Verification items for this drawing (mm, ordinates from the low corner). Coordinates: 2 decimals unless noted, no trailing zeros. Order: outer loops, then holes, each group sorted by start corner. A loop starts at its lowest first (then second) coordinate and runs counter-clockwise, first axis right, second up.
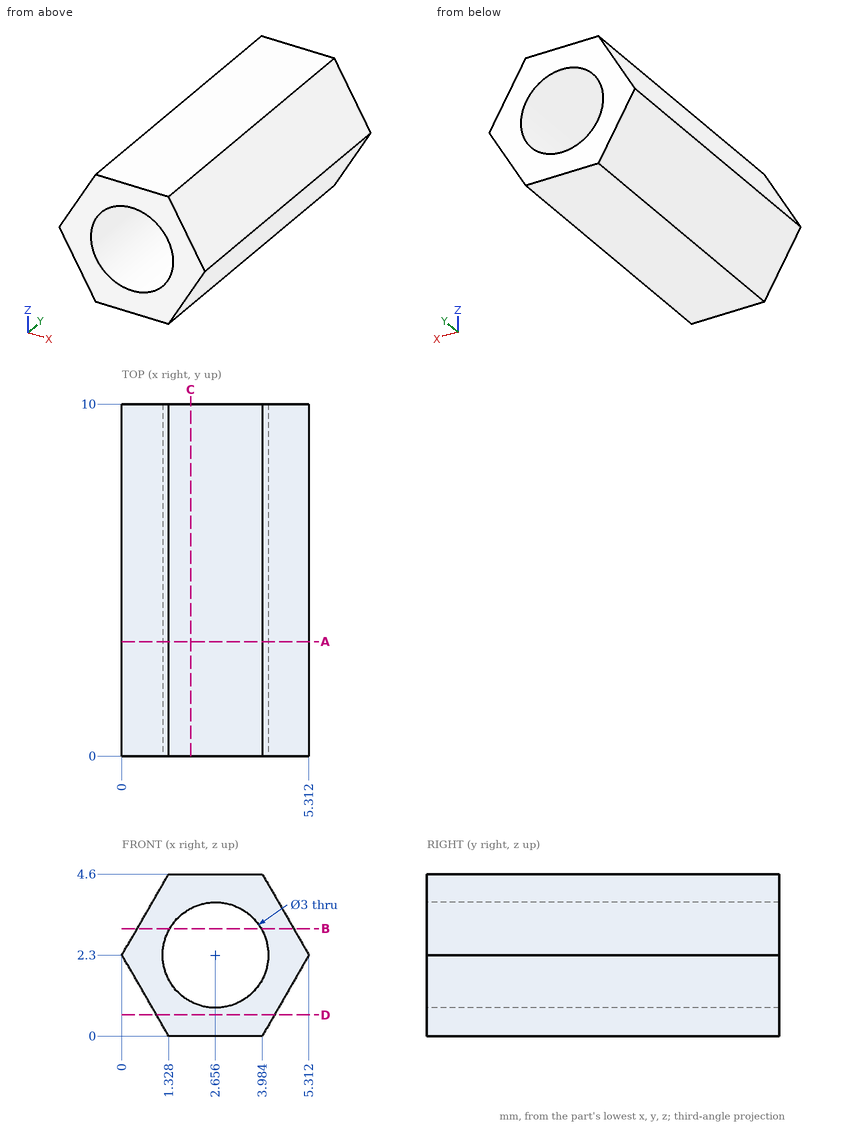
Item 1: Sectioned sample at D-D (z = 0.6). Record the cut outline in (x, y).
Item 2: Thickness scan on line 1 along Z through (x, y) = (2, 3.75); line 2 along Z through (x, y) = (3.5, 4); line 3 along X through (y, z) = (5.5, 1.25) (1 decimal). Record the ranges inside material, lowest first.
Item 3: Sectioned sample at B-B (z = 3.05). Record the cut outline in (x, y) (1 decimal).
Item 4: Sectioned sample at C-C (x = 1.95). Record the cut outline in (y, z).
Item 5: Sectioned sample at A-A (y = 3.25). Record the cut outline in (x, z).
Geometry check:
1. outline: (0.98, 0) - (4.33, 0) - (4.33, 10) - (0.98, 10) - close
2. line 1: z = 0 to 0.95, 3.65 to 4.6
2. line 2: z = 0 to 1.06, 3.54 to 4.6
2. line 3: x = 0.6 to 1.6, 3.7 to 4.7
3. outline: (0.4, 0) - (1.4, 0) - (1.4, 10) - (0.4, 10) - close; (4, 0) - (4.9, 0) - (4.9, 10) - (4, 10) - close
4. outline: (0, 0) - (10, 0) - (10, 0.98) - (0, 0.98) - close; (0, 3.62) - (10, 3.62) - (10, 4.6) - (0, 4.6) - close
5. outline: (0, 2.3) - (1.33, 0) - (3.98, 0) - (5.31, 2.3) - (3.98, 4.6) - (1.33, 4.6) - close; hole circle Ø3 at (2.66, 2.3)
